Work out the finished part from the listing and answer in its coordinate system (mm). A direction names the side the tool comes from. Coordinates: 2 decimals unless noted, no trailing zeros. Loops run counter-clockwise (first coordinate to the right, second up) from the corner with the lowest first, then second, coordinate; pieces in that order, holes last. Notation, with made-up numbers: M 75.5,24.25 L 95.5,24.25 A27 ccw 95.5,46.25 Z; hole C 72,15.5 d9. An arc over 180 degrees is marked long. Write each question's results on one line, items separated by ' | '.
```python
from build123d import *

# Parameters (mm, degrees)
SZKIC1_W                            = 200
SZKIC1_H                            = 20
DODANIE_WYCI_GNI_CIE1_DEPTH         = 7
OTWORY_USTALAJ_CE_8_0MM1_AT_2_COUNT = 2
OTWORY_USTALAJ_CE_8_0MM1_AT_2_PITCH = 90
OTWORY_USTALAJ_CE_8_0MM1_AT_3_COUNT = 2
OTWORY_USTALAJ_CE_8_0MM1_AT_3_PITCH = 180


with BuildPart() as part:
    # Szkic1 → Dodanie-wyciągnięcie1 (new body)
    with BuildSketch(Plane(origin=(0, 0, 0), x_dir=(1, 0, 0), z_dir=(0, 1, 0))):
        Rectangle(SZKIC1_W, SZKIC1_H)
        with BuildLine():
            Line((-75, 5), (-15, 5))
            ThreePointArc((-15, 5), (-10, 0), (-15, -5))
            Line((-15, -5), (-75, -5))
            ThreePointArc((-75, -5), (-80, 0), (-75, 5))
        make_face(mode=Mode.SUBTRACT)
        with BuildLine():
            Line((75, 5), (15, 5))
            ThreePointArc((15, 5), (10, 0), (15, -5))
            Line((15, -5), (75, -5))
            ThreePointArc((75, -5), (80, 0), (75, 5))
        make_face(mode=Mode.SUBTRACT)
    extrude(amount=DODANIE_WYCI_GNI_CIE1_DEPTH)

    # Szkic4 → Otwory ustalające Ø8.0mm1 (revolve, cut)
    with BuildSketch(Plane(origin=(-90, 7, 0), x_dir=(0, 0, 1), z_dir=(1, 0, 0))):
        Polygon((0, 0), (0, 7), (4.5, 7), (4, 6.5), (4, 0.5), (4.5, 0), align=None)
    otwory_ustalaj_ce_8_0mm1 = revolve(axis=Axis((-90, 13.35, 0), (0, -1, 0)), mode=Mode.SUBTRACT)

    # Otwory ustalające Ø8.0mm1 at 2: Otwory ustalające Ø8.0mm1 ×2
    with Locations(*[(i * OTWORY_USTALAJ_CE_8_0MM1_AT_2_PITCH, 0, 0) for i in range(1, OTWORY_USTALAJ_CE_8_0MM1_AT_2_COUNT)]):
        add(otwory_ustalaj_ce_8_0mm1, mode=Mode.SUBTRACT)

    # Otwory ustalające Ø8.0mm1 at 3: Otwory ustalające Ø8.0mm1 ×2
    with Locations(*[(i * OTWORY_USTALAJ_CE_8_0MM1_AT_3_PITCH, 0, 0) for i in range(1, OTWORY_USTALAJ_CE_8_0MM1_AT_3_COUNT)]):
        add(otwory_ustalaj_ce_8_0mm1, mode=Mode.SUBTRACT)


solid = part.part
```
1) Find section C-C, the plane z = 0. Give the number of separate pieces and of enclosed holes in the cut face, and give its area (4 significant figures).
Check result:
separate pieces: 6 | enclosed holes: 0 | area: 250.5 mm^2
2) Which of the six approach directions +Z, -Z, +X, -X, +Y, -Y give full straight-line access (tool end or side, diameter ignored) to faces 1 (the face through (-1, 3, 10)), 2 (the face through (-45, 3, 5))?
Check result:
face 1: +Z, +X, -X, +Y, -Y | face 2: +Y, -Y
3) Straight lines are drawn through the part: probe 1 along X at (y, z) = (4.85, 0); probe 2 along Z at (x, y) = (90, 2.15); probe 3 along Z at (x, y) = (-65, 6.25). For each, find the intervals that lie inside material, in ascending order. Write a range as [from, to].
Check result:
probe 1: [-100, -94], [-86, -80], [-10, -4], [4, 10], [80, 86], [94, 100] | probe 2: [-10, -4], [4, 10] | probe 3: [-10, -5], [5, 10]
4) Find section D-D, the plane x = 90. Give the vertices of the cut face in (y, z).
Check result:
outline: M 0,-10 L 7,-10 L 7,-4.5 L 6.5,-4 L 0.5,-4 L 0,-4.5 Z; M 0,4.5 L 0.5,4 L 6.5,4 L 7,4.5 L 7,10 L 0,10 Z
5) Find section A-A, the plane x = -37.5. Give the vertices of the cut face in (y, z).
Check result:
outline: M 0,-10 L 7,-10 L 7,-5 L 0,-5 Z; M 0,5 L 7,5 L 7,10 L 0,10 Z
6) Find section B-B, the plane y = 3.75. Give the vertices of the cut face in (x, z), and give its area (3 significant figures).
Check result:
outline: M -100,-10 L 100,-10 L 100,10 L -100,10 Z; hole C -90,0 d8; hole M -75,-5 L -15,-5 A5 ccw -15,5 L -75,5 A5 ccw Z; hole C 0,0 d8; hole M 15,-5 L 75,-5 A5 ccw 75,5 L 15,5 A5 ccw Z; hole C 90,0 d8 | area: 2,490 mm^2
7) Given pin 1 Ø5 at (x, z) = (-90, 0) entering from +Y, flat-ended and moving along its own axis, determine where the tip first touches the part or whether it passes through.
Check result:
pin 1: through
